Geometry check sheet. Reference: the model listing, model coordinates, mm. Round coordinates to 2 decimals unless told otherwise and drop trailing zeros. Order: outer loops, then holes, each group sorted by start corner. A loop starts at its lowest first (then second) coordinate and runs counter-clockwise, first axis right, second up. Notation, with made-up numbers: (88.25, -17.75) - (113.25, -17.75) arc R32 ccw to (113.25, 21.25) - close; hole circle Ø7 at (-38, 73). An arc over 180 degrees is marked (long way). Return JSON: item names as keys, results as strings. Group by question number.
Q1. Sectioned sample at D-D, the plane x = 126. Record the cut outline in (y, z).
Q2. Sectioned sample at B-B, the plane x = 75. Record the cut outline in (y, z).
Q3. Sectioned sample at C-C, the plane y = -47.5. Record the cut outline in (x, z), then the cut area to 3 significant figures.
Q4. Material ranges on line 1 along X through (y, z) = (-49, 0); line 2 along Z through (x, y) = (23, -46); line 3 along Z through (x, y) = (70.5, -53), recorded low to high.
Q5. Draft check along Z on faces 1 (the cylindrical face through (52.46, -49.13, -0.9)), 2 (the cylindrical face through (73.95, -49.368, -51.027)), 3 (the flat face through (76, -54.2, 11)). Enter one of: pulls with the +Z half, pulls with the -Z half, needs draft (parallel to the pull), parting line crosses it, or undercut.
Q6. Sectioned sample at A-A, the plane z = 0. Record the cut outline in (x, y).
Autodesk Inventor part; units mm, degrees
ref_plane "YZ Plane" through (0, 0, 0) normal (1, 0, 0) x (0, 1, 0)
ref_plane "XZ Plane" through (0, 0, 0) normal (0, 1, 0) x (-1, 0, 0)
ref_plane "XY Plane" through (0, 0, 0) normal (0, 0, 1) x (1, 0, 0)
sketch "Sketch1" plane through (0, 0, 0) normal (1, 0, 0) x (0, 1, 0)
  circle A0 centre (0, 0) radius 71
  dimension "d0" = 142
extrude "Extrusion1" add sketch "Sketch1" along normal blind 150
sketch "Sketch2" plane through (150, 0, 0) normal (1, 0, 0) x (0, 0, -1)
  line L0 (0, 0) -> (0, -44.2)
  circle A0 centre (0, 0) radius 71
  line L1 (-55.564, -44.2) -> (55.564, -44.2)
  dimension "d3" = 44.2
extrude "Extrusion2" cut sketch "Sketch2" against normal blind 150 contours A0 L1 picked at (-0.2063, 32.437)
sketch "Sketch3" plane through (150, 0, 0) normal (1, 0, 0) x (0, 0, -1)
  line L0 (0, 0) -> (0, -54.2)
  arc A0 (-55.564, -44.2) -> (55.564, -44.2) centre (0, 0) ccw
  line L1 (-45.8624, -54.2) -> (45.8624, -54.2)
  dimension "d6" = 54.2
extrude "Extrusion3" cut sketch "Sketch3" against normal blind 150
sketch "Sketch6" plane through (150, -44.2, 55.564) normal (0, 1, 0) x (1, 0, 0)
  line L0 (-150, 55.564) -> (-75, 55.564)
  circle A0 centre (-75, 55.564) radius 3
  line L1 (-75, 55.564) -> (-49.6, 55.564)
  line L2 (-49.6, 55.564) -> (-24.2, 55.564)
  line L3 (-75, 55.564) -> (-100.4, 55.564)
  line L4 (-100.4, 55.564) -> (-125.8, 55.564)
  circle A1 centre (-100.4, 55.564) radius 3
  circle A2 centre (-125.8, 55.564) radius 3
  circle A3 centre (-24.2, 55.564) radius 3
  circle A4 centre (-49.6, 55.564) radius 3
  dimension "d51" = 75
  dimension "d52" = 6
  dimension "d53" = 25.4
  dimension "d54" = 25.4
  dimension "d55" = 25.4
  dimension "d56" = 25.4
  dimension "d57" = 6
  dimension "d58" = 6
  dimension "d59" = 6
  dimension "d60" = 6
extrude "Extrusion4" cut sketch "Sketch6" against normal blind 10
thread "Thread1"
thread "Thread2"
thread "Thread3"
thread "Thread4"
properties part number "Base"
Reply:
{
 "1": {"outline": "(-54.2, -45.86) arc R71 ccw to (-44.2, -55.56) - (-44.2, -2.99) - (-54.2, -2.99) - close; (-54.2, 2.99) - (-44.2, 2.99) - (-44.2, 55.56) arc R71 ccw to (-54.2, 45.86) - close"},
 "2": {"outline": "(-54.2, -45.86) arc R71 ccw to (-44.2, -55.56) - (-44.2, -3) - (-54.2, -3) - close; (-54.2, 3) - (-44.2, 3) - (-44.2, 55.56) arc R71 ccw to (-54.2, 45.86) - close"},
 "3": {"outline": "(0, -52.77) - (150, -52.77) - (150, 52.77) - (0, 52.77) - close; hole circle Ø6 at (24.2, 0); hole circle Ø6 at (49.6, 0); hole circle Ø6 at (75, 0); hole circle Ø6 at (100.4, 0); hole circle Ø6 at (125.8, 0)", "area": "15,700 mm^2"},
 "4": {"line 1": "0 to 21.2, 27.2 to 46.6, 52.6 to 72, 78 to 97.4, 103.4 to 122.8, 128.8 to 150", "line 2": "-54.08 to -2.75, 2.75 to 54.08", "line 3": "-47.24 to 47.24"},
 "5": {"face 1": "undercut", "face 2": "pulls with the -Z half", "face 3": "needs draft"},
 "6": {"outline": "(0, -54.2) - (21.2, -54.2) - (21.2, -44.2) - (0, -44.2) - close; (27.2, -54.2) - (46.6, -54.2) - (46.6, -44.2) - (27.2, -44.2) - close; (52.6, -54.2) - (72, -54.2) - (72, -44.2) - (52.6, -44.2) - close; (78, -54.2) - (97.4, -54.2) - (97.4, -44.2) - (78, -44.2) - close; (103.4, -54.2) - (122.8, -54.2) - (122.8, -44.2) - (103.4, -44.2) - close; (128.8, -54.2) - (150, -54.2) - (150, -44.2) - (128.8, -44.2) - close"}
}
